Build history of the part. All positions in model axes, mm. A direction names the side the tool comes from. Give positions to 0.01 mm unless a question says otherwise; leave off trailing zeros. Write each loop counter-clockwise with the first axis right and the second up, starting at its lowest first coordinate (ties: lowest second). Pieces come first, ordered by that corner, then holes. Notation, with made-up numbers: (56.5, -11.75) -> (103.5, -11.75) arc R31 cw to (103.5, 15.25) -> close; hole circle Ø2 at (75.25, 88). An arc over 180 degrees is marked (long way). Put each result on its own line as item: value.
from build123d import *

# Parameters (mm, degrees)
F0_W     = 58.18182
F0_H     = 109.090917
F0_W_2   = 30.922429
F0_H_2   = 85.915956
F1_DEPTH = 15
F3_D     = 5.5


with BuildPart() as f1:
    # F0 (on Top) → F1 (new body)
    with BuildSketch(Plane.XY):
        with Locations((-9.090909, -9.431821)):
            Rectangle(F0_W, F0_H)
        with Locations((-7.289599, -6.676143)):
            Rectangle(F0_W_2, F0_H_2, mode=Mode.SUBTRACT)
    extrude(amount=F1_DEPTH)

    # F3 (through all)
    with Locations(Plane(origin=(-38.181819, 0, 0), x_dir=(0, -1, 0), z_dir=(-1, 0, 0))):
        with Locations((-27.727274, 3.977273), (40.68182, 3.977273)):
            Hole(F3_D / 2)


solid = f1.part
1) Tool access for faces 1 (the flat face through (-22.751, -7, 7)), 2 (the cylindrical face through (-30.358, -38.059, 4.803)): list every direction of +Z, -Z, +X, -X, +Y, -Y with a clear straight run to the whole face (end or side of a thin tool).
Filled sheet:
face 1: +Z, -Z
face 2: +X, -X
2) Slice it at D-D (x = -28.5). Write the cut outline in (y, z).
Filled sheet:
outline: (-63.98, 0) -> (45.11, 0) -> (45.11, 15) -> (-63.98, 15) -> close; hole circle Ø5.5 at (-40.68, 3.98); hole circle Ø5.5 at (27.73, 3.98)
3) Slice it at B-B (y = 2.5). Write the cut outline in (x, z).
Filled sheet:
outline: (-38.18, 0) -> (-22.75, 0) -> (-22.75, 15) -> (-38.18, 15) -> close; (8.17, 0) -> (20, 0) -> (20, 15) -> (8.17, 15) -> close
4) Pull direction Z, two halves, no side cores. Call faces 3 (the flat face through (8.172, -7, 7)), 4 (the flat face through (-29, -9, 15)), 5 (the cylindrical face through (14.169, -38.059, 4.803)), 6 (the cylindrical face through (14.17, 30.35, 4.8)): released by +Z, released by -Z, zero draft, split by the parting line, or undercut.
Filled sheet:
face 3: zero draft
face 4: released by +Z
face 5: undercut
face 6: undercut
5) Slice it at A-A (x = -15). Write the cut outline in (y, z), plus the area to 3 significant figures.
Filled sheet:
outline: (-63.98, 0) -> (-49.63, 0) -> (-49.63, 15) -> (-63.98, 15) -> close; (36.28, 0) -> (45.11, 0) -> (45.11, 15) -> (36.28, 15) -> close
area: 348 mm2
6) Slice it at C-C (z = 9). Write the cut outline in (x, y), plus the area to 3 significant figures.
Filled sheet:
outline: (-38.18, -63.98) -> (20, -63.98) -> (20, 45.11) -> (-38.18, 45.11) -> close; hole (-22.75, -49.63) -> (8.17, -49.63) -> (8.17, 36.28) -> (-22.75, 36.28) -> close
area: 3,690 mm2
7) Wall check: L1, parallel to X at y = 3.5, z = 5.75; L2, parallel to Y at x = -17, z = 4.5; L3, parallel to Y at x = 12.5, z = 3.5. Give the ranges that are in metal, low to high.
Filled sheet:
L1: -38.18 to -22.75, 8.17 to 20
L2: -63.98 to -49.63, 36.28 to 45.11
L3: -63.98 to -43.39, -37.97 to 25.02, 30.44 to 45.11
8) Pin check, flat tip, straight feed: pin 1 (5 mm diameter, centred on y = 27.73, z = 3.98, fed in from +X). Stop position of the tip, or through.
Filled sheet:
pin 1: through
